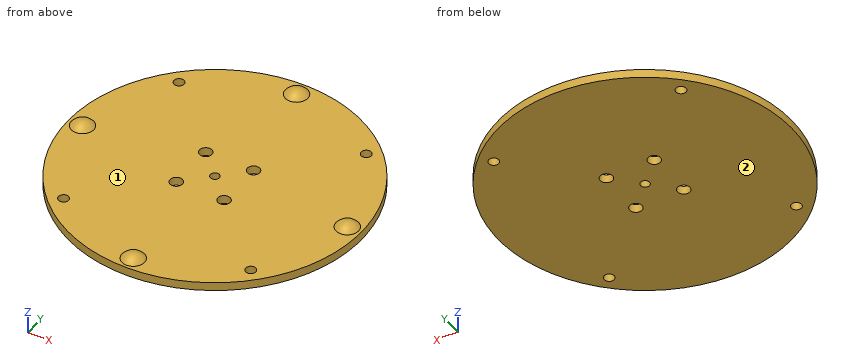
from build123d import *

# Parameters (mm, degrees)
SKETCH004_R             = 52
SKETCH004_R_2           = 1.6
SKETCH004_R_3           = 2.2
PAD003_DEPTH            = 3
SKETCH006_R             = 1.8
POCKET001_DEPTH         = 0.001
POCKET001_DEPTH_BACK    = 3.001
BODY002_PLACEMENT_ANGLE = 180


with BuildPart() as part:
    # Sketch004 → Pad003 (new body)
    with BuildSketch(Plane.XY):
        Circle(SKETCH004_R)
        Circle(SKETCH004_R_2, mode=Mode.SUBTRACT)
        with Locations((8.485281, 8.485281)):
            Circle(SKETCH004_R_3, mode=Mode.SUBTRACT)
        with Locations((-8.485281, 8.485281)):
            Circle(SKETCH004_R_3, mode=Mode.SUBTRACT)
        with Locations((-8.485281, -8.485281)):
            Circle(SKETCH004_R_3, mode=Mode.SUBTRACT)
        with Locations((8.485281, -8.485281)):
            Circle(SKETCH004_R_3, mode=Mode.SUBTRACT)
    extrude(amount=PAD003_DEPTH)

    # Sketch006 → Pocket001 (cut, two sides)
    with BuildSketch(Plane.XY) as pocket001_sk:
        with Locations((-33.234019, 33.234019)):
            Circle(SKETCH006_R)
        with Locations((-33.234019, -33.234019)):
            Circle(SKETCH006_R)
        with Locations((33.234019, -33.234019)):
            Circle(SKETCH006_R)
        with Locations((33.234019, 33.234019)):
            Circle(SKETCH006_R)
    extrude(amount=-POCKET001_DEPTH, mode=Mode.SUBTRACT)
    extrude(pocket001_sk.sketch, amount=POCKET001_DEPTH_BACK, mode=Mode.SUBTRACT)

    # Sphere → Sphere (revolve)
    with BuildSketch(Plane.XZ.offset(-47)):
        with BuildLine():
            ThreePointArc((5, 0), (3.535534, 3.535534), (0, 5))
            Line((0, 5), (0, 0))
            Line((0, 0), (5, 0))
        make_face()
    revolve(axis=Axis((0, 47, 0), (0, 0, 1)))

    # Sphere001 → Sphere001 (revolve)
    with BuildSketch(Plane.XZ.offset(47)):
        with BuildLine():
            ThreePointArc((5, 0), (3.535534, 3.535534), (0, 5))
            Line((0, 5), (0, 0))
            Line((0, 0), (5, 0))
        make_face()
    revolve(axis=Axis((0, -47, 0), (0, 0, 1)))

    # Sphere002 → Sphere002 (revolve)
    with BuildSketch(Plane(origin=(47, 0, 0), x_dir=(1, 0, 0), z_dir=(0, -1, 0))):
        with BuildLine():
            ThreePointArc((5, 0), (3.535534, 3.535534), (0, 5))
            Line((0, 5), (0, 0))
            Line((0, 0), (5, 0))
        make_face()
    revolve(axis=Axis((47, 0, 0), (0, 0, 1)))

    # Sphere003 → Sphere003 (revolve)
    with BuildSketch(Plane(origin=(-47, 0, 0), x_dir=(1, 0, 0), z_dir=(0, -1, 0))):
        with BuildLine():
            ThreePointArc((5, 0), (3.535534, 3.535534), (0, 5))
            Line((0, 5), (0, 0))
            Line((0, 0), (5, 0))
        make_face()
    revolve(axis=Axis((-47, 0, 0), (0, 0, 1)))


with BuildPart() as part_1:
    # Body002 placement: moved
    add(part.part.moved(Location((0, 0, 51))).rotate(Axis((0, 0, 51), (0, 0, -1)), BODY002_PLACEMENT_ANGLE))


solid = part_1.part
Can you work these out from the model? Positions are in its coordinate system, mm. Face numbers are marked on the shaded views. A direction names the side the tool comes from. Coordinates: 2 decimals unless noted, no trailing zeros. Order: outer loops, then holes, each group sorted by start corner. A loop starts at its lowest first (then second) coordinate and runs counter-clockwise, first axis right, second up. Notation, with made-up numbers: (67.5, 13) - (87.5, 13) arc R10 ccw to (87.5, 28) - close; hole circle Ø9 at (51, 3.5). An arc over 180 degrees is marked (long way). Answer as a JSON object with one key per item and string values. Group by question number.
Q1. On a 3-axis mill with a long thin cutter (end or side, diameter ignored), from which of +Z, -Z, +X, -X, +Y, -Y can I reach the whole of each face in a straight line? I mean the marked faces 1 and 2. Say none if no direction works.
Q2. Imagine slicing it at B-B (x = -12). Please give me the cut outline in (y, z).
Q3. Will these pins go through, and if not, where does the flat tip stop? P1, Ø2, axis at x = 37, z = 53.5, coming from the -Y side; P2, Ø5, axis at x = -8.49, y = -8.49, coming from the +Z side; P3, Ø3, axis at y = 29.5, z = 53, coming from the +X side.
Q4. Imagine slicing it at A-A (z = 53). Give the number of separate pieces and of enclosed holes in the cut face, and give its area (3 significant figures).
Q5. Imagine slicing it at C-C (y = 38). Please give me the cut outline in (x, z), and give its area (3 significant figures).
Q6. I need wall thicknesses on line 1 (Y direction, x = 0, z = 53.45); line 2 (Y direction, x = -10.5, z = 52.55). Which ranges of each line are inside material? Lowest first, please. Write a range as from..to.
Determined:
{
 "1": {"face 1": "+Z", "face 2": "-Z, +X, -X, +Y, -Y"},
 "2": {"outline": "(-50.6, 51) - (50.6, 51) - (50.6, 54) - (-50.6, 54) - close"},
 "3": {"P1": "stops at y = -37.52", "P2": "stops at z = 54", "P3": "stops at x = 43.82"},
 "4": {"separate pieces": "1", "enclosed holes": "9", "area": "8,390 mm2"},
 "5": {"outline": "(-35.5, 51) - (35.5, 51) - (35.5, 54) - (-35.5, 54) - close", "area": "213 mm2"},
 "6": {"line 1": "y = -52..-1.6, 1.6..52", "line 2": "y = -50.93..-9.37, -7.6..7.6, 9.37..50.93"}
}
